```python
from build123d import *

# Parameters (mm, degrees)
SKETCH1_W               = 56
SKETCH1_H               = 4
BOSS_EXTRUDE1_DEPTH     = 168
SKETCH2_W               = 4
SKETCH2_H               = 18
BOSS_EXTRUDE3_DEPTH     = 4
LPATTERN1_COUNT         = 4
LPATTERN1_PITCH         = 50
MIRROR1_COPY_1_SKETCH_W = 4
MIRROR1_COPY_1_SKETCH_H = 18
MIRROR1_COPY_1_DEPTH    = 4
MIRROR1_COPY_2_SKETCH_W = 4
MIRROR1_COPY_2_SKETCH_H = 18
MIRROR1_COPY_2_DEPTH    = 4
MIRROR1_COPY_3_SKETCH_W = 4
MIRROR1_COPY_3_SKETCH_H = 18
MIRROR1_COPY_3_DEPTH    = 4
SKETCH3_W               = 12
SKETCH3_H               = 4
BOSS_EXTRUDE4_DEPTH     = 4


with BuildPart() as part:
    # Sketch1 → Boss-Extrude1 (new body)
    with BuildSketch(Plane(origin=(0, 0, 0), x_dir=(1, 0, 0), z_dir=(0, 1, 0))):
        Rectangle(SKETCH1_W, SKETCH1_H)
    extrude(amount=BOSS_EXTRUDE1_DEPTH)

    # Sketch2 → Boss-Extrude3 (add, through all)
    with BuildSketch(Plane.XY.offset(2)):
        with Locations((-30, 9)):
            Rectangle(SKETCH2_W, SKETCH2_H)
    boss_extrude3 = extrude(amount=-BOSS_EXTRUDE3_DEPTH)

    # LPattern1: Boss-Extrude3 ×4
    with Locations(*[(0, i * LPATTERN1_PITCH, 0) for i in range(1, LPATTERN1_COUNT)]):
        add(boss_extrude3)

    # Mirror1: Boss-Extrude3 across plane
    add(boss_extrude3.mirror(Plane(origin=(0, 0, 0), x_dir=(0, 0, 1), z_dir=(1, 0, 0))))

    # Mirror1 copy 1 sketch → Mirror1 copy 1 (add, through all)
    with BuildSketch(Plane(origin=(0, 50, 2), x_dir=(-1, 0, 0), z_dir=(0, 0, 1))):
        with Locations((-30, -9)):
            Rectangle(MIRROR1_COPY_1_SKETCH_W, MIRROR1_COPY_1_SKETCH_H)
    extrude(amount=-MIRROR1_COPY_1_DEPTH)

    # Mirror1 copy 2 sketch → Mirror1 copy 2 (add, through all)
    with BuildSketch(Plane(origin=(0, 100, 2), x_dir=(-1, 0, 0), z_dir=(0, 0, 1))):
        with Locations((-30, -9)):
            Rectangle(MIRROR1_COPY_2_SKETCH_W, MIRROR1_COPY_2_SKETCH_H)
    extrude(amount=-MIRROR1_COPY_2_DEPTH)

    # Mirror1 copy 3 sketch → Mirror1 copy 3 (add, through all)
    with BuildSketch(Plane(origin=(0, 150, 2), x_dir=(-1, 0, 0), z_dir=(0, 0, 1))):
        with Locations((-30, -9)):
            Rectangle(MIRROR1_COPY_3_SKETCH_W, MIRROR1_COPY_3_SKETCH_H)
    extrude(amount=-MIRROR1_COPY_3_DEPTH)

    # Sketch3 → Boss-Extrude4 (add, through all)
    with BuildSketch(Plane(origin=(0, 0, -2), x_dir=(-1, 0, 0), z_dir=(0, 0, -1))):
        with Locations((26, -2)):
            Rectangle(SKETCH3_W, SKETCH3_H)
        with Locations((0, -2)):
            Rectangle(SKETCH3_W, SKETCH3_H)
        with Locations((-26, -2)):
            Rectangle(SKETCH3_W, SKETCH3_H)
    boss_extrude4 = extrude(amount=-BOSS_EXTRUDE4_DEPTH)

    # Mirror2: Boss-Extrude4 across plane
    add(boss_extrude4.mirror(Plane(origin=(0, 84, 0), x_dir=(0, 0, 1), z_dir=(0, -1, 0))))


solid = part.part
```
Work out the finished part from the listing and answer in its coordinate system (mm). A direction names the side the tool comes from. Round coordinates to 2 decimals unless told otherwise and drop trailing zeros. Order: outer loops, then holes, each group sorted by start corner. A loop starts at its lowest first (then second) coordinate and runs counter-clockwise, first axis right, second up.
Q1. A cutting plane is placed at A-A, the plane y = 142.5. Determine the outline of the cut face in (x, z), then the cut area to 3 significant figures.
Solution:
outline: (-28, -2) - (28, -2) - (28, 2) - (-28, 2) - close
area: 224 mm2
Q2. The mould has two halves that part along Y. Classify faces 5 (the flat face through (-13, 0, 0)), 6 (the flat face through (30, 18, 0)), 7 (the flat face through (20, -2, 0)): pulls with the +Y half, pulls with the -Y half, needs draft (parallel to the pull), parting line crosses it, or undercut.
Solution:
face 5: pulls with the -Y half
face 6: undercut
face 7: needs draft
Q3. Find the intervals of material crossed by line 1 along X through (y, z) = (98.5, 1.3); line 2 along Y through (x, z) = (-16, 1.3), in increasing order.
Solution:
line 1: x = -28 to 28
line 2: y = 0 to 168
Q4. A tool of negligible diameter and unlimited length cuts with its end or side. For faces 1 (the flat face through (30, 100, 0)), 2 (the flat face through (-13, 168, 0)), 3 (the flat face through (-30, 68, 0)), 4 (the flat face through (13, 0, 0)), from which of +Z, -Z, +X, -X, +Y, -Y can it reach the whole face along a straight path? Write none if from no direction.
Solution:
face 1: +Z, -Z, +X
face 2: +Z, -Z, +Y
face 3: +Z, -Z, -X
face 4: +Z, -Z, -Y
Q5. A cutting plane is placed at B-B, the plane x = 10.5. Determine the outline of the cut face in (y, z).
Solution:
outline: (0, -2) - (168, -2) - (168, 2) - (0, 2) - close
Q6. Given pin 1 Ø2 at (y, z) = (136, 0.5) entering from -X; pin 2 Ø1.2 at (y, z) = (86, 0) entering from +X; pin 3 Ø2 at (x, z) = (12.5, -1) entering from -Y, each flat-ended and moving along its own axis, determine where each tip first touches the part or whether it passes through.
Solution:
pin 1: stops at x = -28
pin 2: stops at x = 28
pin 3: stops at y = 0
